Autodesk Fusion 360 part; units mm, degrees
sketch "Sketch1" plane through (0, 0, 0) normal (0, 0, 1) x (1, 0, 0)
  line L0 (-15, -21) -> (15, -21)
  line L1 (15, -21) -> (15, 21)
  line L2 (15, 21) -> (-15, 21)
  line L3 (-15, 21) -> (-15, -21)
  line L4 (-15, -21) -> (15, 21) construction
  line L5 (15, -21) -> (-15, 21) construction
  line L6 (0, -21) -> (7, -21) construction
  line L7 (7, -21) -> (7, -9) construction
  line L8 (7, -9) -> (0, -9) construction
  line L9 (0, -9) -> (0, -21) construction
  line L10 (0, -21) -> (-7, -21) construction
  line L11 (-7, -21) -> (-7, -9) construction
  line L12 (-7, -9) -> (0, -9) construction
  line L13 (0, -9) -> (0, -21) construction
  circle A0 centre (-7, -9) radius 4
  circle A1 centre (7, -9) radius 4
  dimension "d1" = 30
  dimension "d2" = 42
  dimension "d3" = 7
  dimension "d4" = 12
  dimension "d5" = 7
  dimension "d6" = 12
  dimension "d7" = 8
  dimension "d8" = 8
extrude "Extrude1" add sketch "Sketch1" along normal blind 5 makes body 1
sketch "Sketch2" plane through (0, 0, 5) normal (0, 0, 1) x (-1, 0, 0)
  circle A0 centre (-7, 9) radius 4
  circle A1 centre (7, 9) radius 4
  line L0 (15, -21) -> (15, 21)
  line L1 (15, 21) -> (-15, 21)
  line L2 (-15, 21) -> (-15, -21)
  line L3 (-15, -21) -> (15, -21)
  line L4 (15, 21) -> (-15, 21)
  line L5 (-15, 21) -> (-15, 19)
  line L6 (-15, 19) -> (15, 19)
  line L7 (15, 19) -> (15, 21)
  dimension "d11" = 30
  dimension "d12" = 2
extrude "Extrude2" add sketch "Sketch2" along normal blind 25 contours L0 L1 L2 L4 L5 L6 L7 bodies 1
sketch "Sketch3" plane through (0, 0, 0) normal (0, 0, -1) x (1, 0, 0)
  circle A0 centre (7, 9) radius 4
  circle A1 centre (-7, 9) radius 4
  line L0 (-15, 21) -> (-15, -21)
  line L1 (-15, -21) -> (15, -21)
  line L2 (15, -21) -> (15, 21)
  line L3 (15, 21) -> (-15, 21)
  line L4 (0, 21) -> (-1.5, 21) construction
  line L5 (-1.5, 21) -> (-1.5, -6) construction
  line L6 (-1.5, -6) -> (0, -6) construction
  line L7 (0, -6) -> (0, 21) construction
  line L8 (0, 21) -> (1.5, 21) construction
  line L9 (1.5, 21) -> (1.5, -6) construction
  line L10 (1.5, -6) -> (0, -6) construction
  line L11 (0, -6) -> (0, 21) construction
  circle A2 centre (0, -6) radius 3.05
  circle A3 centre (-1.5, -6) radius 0.5
  circle A4 centre (1.5, -6) radius 0.5
  dimension "d15" = 1.5
  dimension "d16" = 27
  dimension "d17" = 27
  dimension "d18" = 6.1
  dimension "d19" = 1
  dimension "d20" = 1
extrude "Extrude3" cut sketch "Sketch3" against normal blind 3 contours A2 bodies 1
extrude "Extrude4" cut 2 faces at (1.3037, 5.8866, 0) (-1.4875, 6.1662, 0) along direction (0, 0, -1) up to surface end surface through (0, 0, 5) normal (0, 0, 1) offset 0 on bodies 1 bodies 1
copy_body "Body->Comp1" bodies 1 removing the originals makes body 2 in component "LED_Holder"
component "LED_Holder" placed x (1, 0, 0) y (0, 1, 0) z (0, 0, 1) at (0, 0, 0)
Check sheet for the modelled part. Datum: model origin and axes. Units: mm. A direction names the side the tool comes from. Round coordinates to 2 decimals unless told otherwise and drop trailing zeros. Order: outer loops, then holes, each group sorted by start corner. A loop starts at its lowest first (then second) coordinate and runs counter-clockwise, first axis right, second up. Notation, with made-up numbers: (-16, 53.5) -> (4, 53.5) arc R21 cw to (4, 68.5) -> close; hole circle Ø8 at (62.5, 29.5). An arc over 180 degrees is marked (long way). Use CSV: the item, a comma, the result in double quotes.
(1) Depth check by flat-ended pin: pin 1 (15 mm diameter, centred on x = -2.5, y = 7, fed in from +Z); pin 2 (2 mm diameter, centred on x = -7.5, y = -4.5, fed in from -Z); pin 3 (6 mm diameter, centred on y = 10, z = 10.5, fed in from -X); pin 4 (4 mm diameter, centred on x = -10.5, z = 11.5, fed in from +Y). Enter the tip coordinate at first touch or a pass-through.
Worked out:
pin 1,"z = 5"
pin 2,"z = 0"
pin 3,"through"
pin 4,"y = -19"
(2) Cross-section at A-A (y = -9). Record the boundary of the cut face in (x, z), and give its area (3 significant figures).
Worked out:
outline,"(-15, 0) -> (-11, 0) -> (-11, 5) -> (-15, 5) -> close; (-3, 0) -> (3, 0) -> (3, 5) -> (-3, 5) -> close; (11, 0) -> (15, 0) -> (15, 5) -> (11, 5) -> close"
area,"70.0 mm²"
(3) Material ranges on line 1 along X through (y, z) = (6, 3.75); line 2 along Y through (x, z) = (0, 1.15); line 3 along Y through (x, z) = (-1.5, 3.9), recorded low to high. Write a range as from..to.
Worked out:
line 1,"-15..-2, -1..1, 2..15"
line 2,"-21..2.95, 9.05..21"
line 3,"-21..5.5, 6.5..21"
(4) Cross-section at B-B (x = 7). Record the boundary of the cut face in (y, z), and give its area (3 significant figures).
Worked out:
outline,"(-21, 0) -> (-13, 0) -> (-13, 5) -> (-19, 5) -> (-19, 30) -> (-21, 30) -> close; (-5, 0) -> (21, 0) -> (21, 5) -> (-5, 5) -> close"
area,"220 mm²"
(5) Tool access check on faces 4 (the face through (1, 6, 4)), 5 (the face through (0, 6, 3)), 6 (the face through (0, 1, 5)). Record the directions out of +Z, -Z, +X, -X, +Y, -Y that give a thin tool (end or side, any length) a straight path to the whole face; none if there is none.
Worked out:
face 4,"+Z, -Z"
face 5,"-Z"
face 6,"+Z, +X, -X, +Y"
(6) Draft check along Y on faces 1 (the face through (-0.661, 8.977, 1.479)), 2 (the face through (0, -19, 17)), 3 (the face through (15, -3, 4)). Enter one of: pulls with the +Y half, pulls with the -Y half, needs draft (parallel to the pull), parting line crosses it, or undercut.
Worked out:
face 1,"undercut"
face 2,"pulls with the +Y half"
face 3,"needs draft"
(7) Cross-section at D-D (y = 6). Record the boundary of the cut face in (x, z), and give its area (3 significant figures).
Worked out:
outline,"(-15, 0) -> (-3.05, 0) -> (-3.05, 3) -> (-2, 3) -> (-2, 5) -> (-15, 5) -> close; (-1, 3) -> (1, 3) -> (1, 5) -> (-1, 5) -> close; (2, 3) -> (3.05, 3) -> (3.05, 0) -> (15, 0) -> (15, 5) -> (2, 5) -> close"
area,"128 mm²"
(8) Cross-section at C-C (z = 4.5). Record the boundary of the cut face in (x, y).
Worked out:
outline,"(-15, -21) -> (15, -21) -> (15, 21) -> (-15, 21) -> close; hole circle Ø8 at (-7, -9); hole circle Ø1 at (-1.5, 6); hole circle Ø1 at (1.5, 6); hole circle Ø8 at (7, -9)"
